from build123d import *

# Parameters (mm, degrees)
BOSS_EXTRUDE1_DEPTH = 3.175
SKETCH1_4_R         = 3.6
CUT_EXTRUDE1_DEPTH  = 439.905857431
FILLET1_R           = 48
CUT_EXTRUDE3_DEPTH  = 10
CUT_EXTRUDE5_DEPTH  = 10
SKETCH11_R          = 2
CUT_EXTRUDE6_DEPTH  = 10


with BuildPart() as part:
    # Sketch1 → Boss-Extrude1 (new body)
    with BuildSketch(Plane.XY):
        Polygon((428.120588235, 28.939617947), (0.540381846, 28.939617947), (-115.605170134, 28.939617947), (-98.879411765, 3.850980392), (-31.879411765, -96.649019608), (366, -96.649019608), (403.120588235, -71.149019608), align=None)
    extrude(amount=BOSS_EXTRUDE1_DEPTH)

    # Sketch1<4> → Cut-Extrude1 (cut, through all)
    with BuildSketch(Plane.XY):
        with Locations((-12.879411765, -83.899019608)):
            Circle(SKETCH1_4_R)
        with Locations((51.120588235, -83.899019608)):
            Circle(SKETCH1_4_R)
        with Locations((115.120588235, -83.899019608)):
            Circle(SKETCH1_4_R)
        with Locations((179.120588235, -83.899019608)):
            Circle(SKETCH1_4_R)
        with Locations((243.120588235, -83.899019608)):
            Circle(SKETCH1_4_R)
        with Locations((307.120588235, -83.899019608)):
            Circle(SKETCH1_4_R)
    extrude(amount=CUT_EXTRUDE1_DEPTH, mode=Mode.SUBTRACT)

    # Fillet1
    fillet1_edges = [part.edges().sort_by_distance(p)[0] for p in [
        (-31.879411765, -96.649019608, 1.5875),
    ]]
    fillet(fillet1_edges, radius=FILLET1_R)

    # Sketch7 → Cut-Extrude3 (cut)
    with BuildSketch(Plane.XY.offset(3.175)):
        Polygon((403.120588235, -71.149019608), (340.005873473, -96.649019608), (366, -96.649019608), align=None)
    extrude(amount=-CUT_EXTRUDE3_DEPTH, mode=Mode.SUBTRACT)

    # Sketch10 → Cut-Extrude5 (cut)
    with BuildSketch(Plane.XY.offset(3.175)):
        Polygon((-49.086078431, -70.839019608), (403.198019602, -70.839019608), (428.120588235, 28.939617947), (-115.605170134, 28.939617947), align=None)
    extrude(amount=-CUT_EXTRUDE5_DEPTH, mode=Mode.SUBTRACT)

    # Sketch11 → Cut-Extrude6 (cut)
    with BuildSketch(Plane.XY.offset(3.175)):
        with Locations((-3.879411765, -83.899019608)):
            Circle(SKETCH11_R)
        with Locations((10.120588235, -83.899019608)):
            Circle(SKETCH11_R)
        with Locations((60.120588235, -83.899019608)):
            Circle(SKETCH11_R)
        with Locations((74.120588235, -83.899019608)):
            Circle(SKETCH11_R)
        with Locations((124.120588235, -83.899019608)):
            Circle(SKETCH11_R)
        with Locations((138.120588235, -83.899019608)):
            Circle(SKETCH11_R)
        with Locations((188.120588235, -83.899019608)):
            Circle(SKETCH11_R)
        with Locations((202.120588235, -83.899019608)):
            Circle(SKETCH11_R)
        with Locations((252.120588235, -83.899019608)):
            Circle(SKETCH11_R)
        with Locations((266.120588235, -83.899019608)):
            Circle(SKETCH11_R)
        with Locations((316.120588235, -83.899019608)):
            Circle(SKETCH11_R)
        with Locations((330.120588235, -83.899019608)):
            Circle(SKETCH11_R)
    extrude(amount=-CUT_EXTRUDE6_DEPTH, mode=Mode.SUBTRACT)


solid = part.part
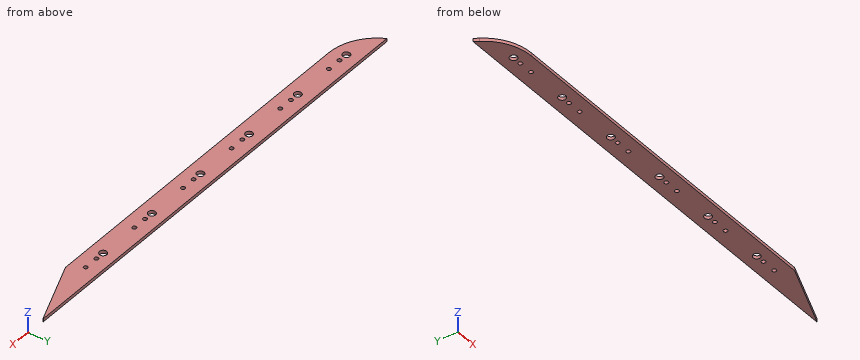
The listing builds one solid part. Answer for the finished solid, in the listing's coordinates (mm). Round coordinates to 2 decimals unless told otherwise and drop trailing zeros. Write each loop counter-clockwise with the first axis right and the second up, starting at its lowest first coordinate (ties: lowest second). Pieces come first, ordered by that corner, then holes. Notation, with made-up numbers: (4, 7) - (11, 7) arc R34 ccw to (11, 38) - close; hole circle Ø10 at (41, 78.25). An arc over 180 degrees is marked (long way). Use a Markdown table: item, result. Add a question column.
1. The part is cut by section B-B (y = -93). Write down the section's boundary in (x, z) (3 decimals).
2. A flat-ended cylindrical pin translates along its axis: P1, Ø4.5, axis at x = -12.88, y = -83.9, coming from the +Z side. Find the tip coordinate at first contact, or state that the pin passes through.
3. The part is cut by section A-A (z = 1.15). Give the number of separate pieces and of enclosed holes in the cut face, and give its area (3 significant figures).
4. Consider line 1 (Y direction, x = 315.5, z = 1.4); line 2 (Y direction, x = 251, z = 1.15); line 3 (X direction, y = -92, z = 1.25). Determine where each line is inside the solid, lowest interval first.
5. The part is cut by section C-C (x = 371). Write down the section's boundary in (y, z) (3 decimals).
Reported:
| question | item | result |
|---|---|---|
| 1 | outline | (-24.548, 0) - (349.038, 0) - (349.038, 3.175) - (-24.548, 3.175) - close |
| 2 | P1 | through |
| 3 | separate pieces | 1 |
| 3 | enclosed holes | 18 |
| 3 | area | 10,100 mm^2 |
| 4 | line 1 | -96.65 to -85.8, -82 to -70.84 |
| 4 | line 2 | -96.65 to -85.56, -82.24 to -70.84 |
| 4 | line 3 | -26.8 to 351.51 |
| 5 | outline | (-84.127, 0) - (-70.839, 0) - (-70.839, 3.175) - (-84.127, 3.175) - close |
